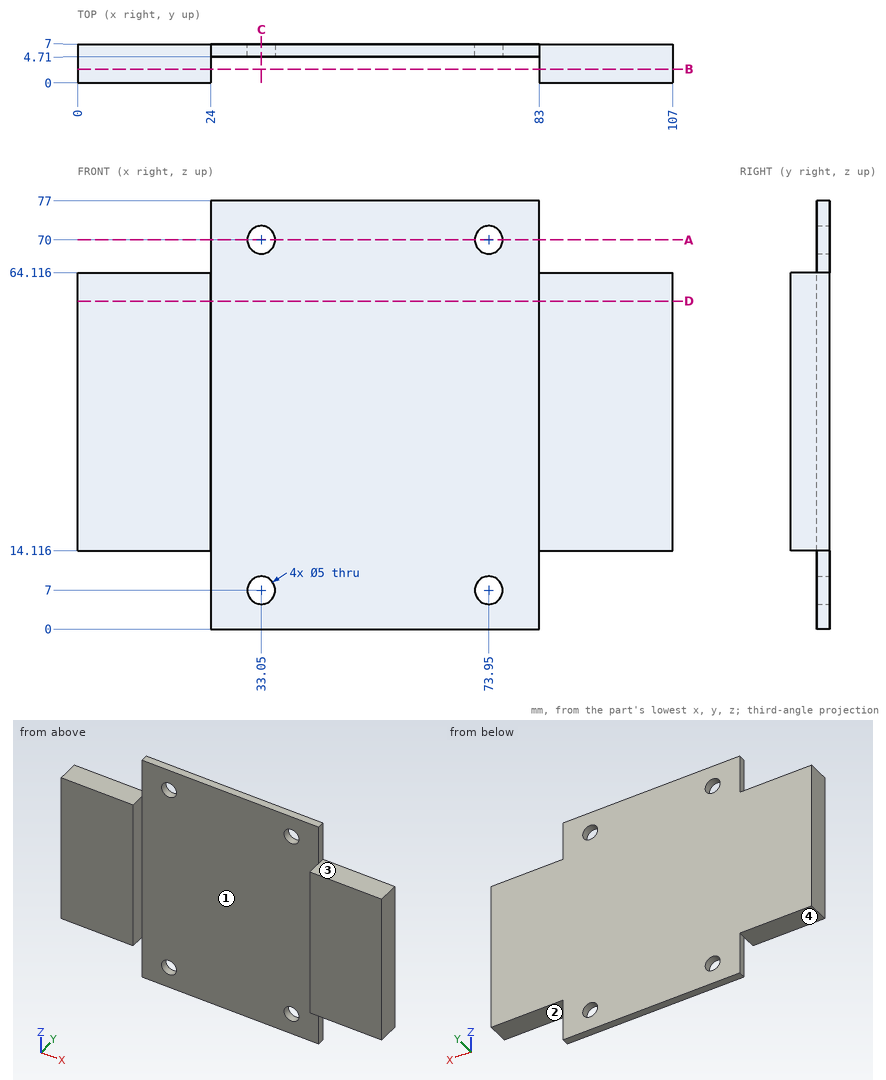
Part print with two shaded views. Sizes in mm from the minimum x, y, z corner. A direction names the side the tool comes from. Coordinates: 2 decimals unless noted, no trailing zeros. Order: outer loops, then holes, each group sorted by start corner. A loop starts at its lowest first (then second) coordinate and runs counter-clockwise, first axis right, second up. Notation, with made-up numbers: (53.25, -16.75) - (103.25, -16.75) arc R23 ccw to (103.25, 21.25) - close; hole circle Ø2 at (17, 27.25). An arc over 180 degrees is marked (long way). Write item = value, one per line. Start each with the question number.
1) 3-axis set-ups, long thin cutter, end or side, ignore diameter. For the marked faces 1, 2, 3 and 4: which of +Z, -Z, +X, -X, +Y, -Y reach the whole face in a straight line?
2) Flat gauge pins, fed straight in: pin 1 Ø8 at (x, z) = (73.95, 7) entering from -Y; pin 2 Ø4 at (x, z) = (73.95, 70) entering from +Y; pin 3 Ø4 at (y, z) = (4.5, 8.5) entering from -X; pin 4 Ø2 at (x, y) = (18, 3) entering from -Z. Where does each tip first touch, or does it go through?
3) Saw through at A-A on z = 70. Write the cut outline in (x, y).
4) Saw through at B-B on y = 2.5. Write the cut outline in (x, z).
5) Saw through at C-C on x = 33.05. Write the cut outline in (y, z), then the cut area to 3 significant figures.
6) Wall check: line 1 along Z through (x, y) = (73.95, 5.7); line 2 along X through (y, z) = (5.85, 70); line 3 along X through (y, z) = (4.5, 46). Give the ranges that are in metal, low to high. Write a range as from..to.
7) Saw through at D-D on z = 59. Write the cut outline in (x, y).
From the geometry:
q1.face_1 = +Z, -Z, -Y
q1.face_2 = -Z, +X, +Y, -Y
q1.face_3 = +Z, +X, +Y, -Y
q1.face_4 = -Z, -X, +Y, -Y
q2.pin_1 = 4.71
q2.pin_2 = through
q2.pin_3 = 24
q2.pin_4 = 14.12
q3.outline = (24, 4.71) - (30.55, 4.71) - (30.55, 7) - (24, 7) - close; (35.55, 4.71) - (71.45, 4.71) - (71.45, 7) - (35.55, 7) - close; (76.45, 4.71) - (83, 4.71) - (83, 7) - (76.45, 7) - close
q4.outline = (0, 14.12) - (24, 14.12) - (24, 64.12) - (0, 64.12) - close; (83, 14.12) - (107, 14.12) - (107, 64.12) - (83, 64.12) - close
q5.outline = (4.71, 0) - (7, 0) - (7, 4.5) - (4.71, 4.5) - close; (4.71, 9.5) - (7, 9.5) - (7, 67.5) - (4.71, 67.5) - close; (4.71, 72.5) - (7, 72.5) - (7, 77) - (4.71, 77) - close
q5.area = 153 mm^2
q6.line_1 = 0..4.5, 9.5..67.5, 72.5..77
q6.line_2 = 24..30.55, 35.55..71.45, 76.45..83
q6.line_3 = 0..24, 83..107
q7.outline = (0, 0) - (24, 0) - (24, 4.71) - (83, 4.71) - (83, 0) - (107, 0) - (107, 7) - (0, 7) - close
